Autodesk Inventor part; units mm, degrees
ref_plane "YZ Plane" through (0, 0, 0) normal (1, 0, 0) x (0, 1, 0)
ref_plane "XZ Plane" through (0, 0, 0) normal (0, 1, 0) x (-1, 0, 0)
ref_plane "XY Plane" through (0, 0, 0) normal (0, 0, 1) x (1, 0, 0)
sketch "Sketch1" plane through (0, 0, 0) normal (0, 1, 0) x (-1, 0, 0)
  line L0 (6, -1.25) -> (-6, -1.25)
  line L1 (-6, -1.25) -> (-6, 1.25)
  line L2 (-6, 1.25) -> (6, 1.25)
  line L3 (6, 1.25) -> (6, -1.25)
  line L4 (6, -1.25) -> (-6, 1.25) construction
  line L5 (-6, -1.25) -> (6, 1.25) construction
  point P0 (0, 0)
  dimension "d0" = 12
  dimension "d1" = 2.5
extrude "Extrusion1" add sketch "Sketch1" along normal blind 0.5
sketch "Sketch2" plane through (0, 0.5, 0) normal (0, 1, 0) x (1, 0, 0)
  circle A0 centre (-4.2565, 0) radius 0.75
  point P0 (0, 0)
  dimension "d4" = 1.5
extrude "Extrusion2" cut sketch "Sketch2" against normal blind 0.5
sketch "Sketch3" plane through (0, 0.5, 0) normal (0, 1, 0) x (1, 0, 0)
  circle A0 centre (-1.7501, 0) radius 0.75
  circle A1 centre (4.2419, 0) radius 0.75
  circle A2 centre (1.7477, 0) radius 0.75
  point P0 (0, 0)
  dimension "d7" = 1.5
  dimension "d8" = 1.5
  dimension "d9" = 1.5
extrude "Extrusion3" cut sketch "Sketch3" against normal blind 0.5 contours A0
sketch "Sketch7" plane through (0, 0.5, 0) normal (0, 1, 0) x (1, 0, 0)
  circle A0 centre (4.7487, 0) radius 0.15
  point P0 (0, 0)
  dimension "d21" = 0.3
extrude "Extrusion7" cut sketch "Sketch7" against normal blind 2
fillet "Fillet2" radius 0.5 1 edges at (6, 0.25, 1.25)
fillet "Fillet3" radius 0.5 1 edges at (6, 0.25, -1.25)
fillet "Fillet4" radius 0.5 1 edges at (-6, 0.25, 1.25)
fillet "Fillet5" radius 0.5 1 edges at (-6, 0.25, -1.25)
properties part number "stationary arm"
Work out the finished part from the listing and answer in its coordinate system (mm). Give positions to 0.01 mm unless a question says otherwise; leave off trailing zeros. Loops run counter-clockwise (first coordinate to the right, second up) from the corner with the lowest first, then second, coordinate; pieces in that order, holes last. Notation, with made-up numbers: (80.25, 14.5) - (100.25, 14.5) arc R26 cw to (100.25, 37.5) - close; hole circle Ø1 at (-30.75, 77). An arc over 180 degrees is marked (long way). Answer in a Markdown table with one row per item.
(1) A flat-ended cylindrical pin translates along its axis: pin 1 Ø1.2 at (x, z) = (-4.26, 0) entering from +Y. Find the tip coordinate at first contact, or state that the pin passes through.
Results list:
| item | result |
|---|---|
| pin 1 | passes through |
(2) Section A-A (x = 4.75) is taken. Give the vertices of the cut face in (y, z), and give its area (3 significant figures).
Results list:
| item | result |
|---|---|
| outline | (0, -1.25) - (0.5, -1.25) - (0.5, -0.15) - (0, -0.15) - close; (0, 0.15) - (0.5, 0.15) - (0.5, 1.25) - (0, 1.25) - close |
| area | 1.10 mm² |
(3) Consider L1, parallel to X at y = 0.45, z = 0; L2, parallel to X at y = 0.45, z = 0.6; L3, parallel to Z at x = -4, y = 0.2. Determine where each line is inside the solid, lowest interval first. Write a range as [from, to].
Results list:
| item | result |
|---|---|
| L1 | x = [-6, -5.01], [-3.51, -2.5], [-1, 4.6], [4.9, 6] |
| L2 | x = [-6, -4.71], [-3.81, -2.2], [-1.3, 6] |
| L3 | z = [-1.25, -0.7], [0.7, 1.25] |
(4) Section B-B (z = 0) is taken. Give the vertices of the cut face in (x, y), and give its area (3 significant figures).
Results list:
| item | result |
|---|---|
| outline | (-6, 0) - (-5.01, 0) - (-5.01, 0.5) - (-6, 0.5) - close; (-3.51, 0) - (-2.5, 0) - (-2.5, 0.5) - (-3.51, 0.5) - close; (-1, 0) - (4.6, 0) - (4.6, 0.5) - (-1, 0.5) - close; (4.9, 0) - (6, 0) - (6, 0.5) - (4.9, 0.5) - close |
| area | 4.35 mm² |
(5) For a pull along X with two mould halves and no side action, classify faces 1 (the face through (0, 0.5, 0)), 2 (the face through (-5.006, 0.254, -0.033)), 3 (the face through (-1.035, 0.254, -0.225)) as pulls with the +X half, pulls with the -X half, needs draft (parallel to the pull), parting line crosses it, or undercut.
Results list:
| item | result |
|---|---|
| face 1 | needs draft |
| face 2 | undercut |
| face 3 | undercut |
(6) Section C-C (y = 0.3) is taken. Give the vertices of the cut face in (x, z).
Results list:
| item | result |
|---|---|
| outline | (-6, -0.75) arc R0.5 ccw to (-5.5, -1.25) - (5.5, -1.25) arc R0.5 ccw to (6, -0.75) - (6, 0.75) arc R0.5 ccw to (5.5, 1.25) - (-5.5, 1.25) arc R0.5 ccw to (-6, 0.75) - close; hole circle Ø1.5 at (-4.26, 0); hole circle Ø1.5 at (-1.75, 0); hole circle Ø0.3 at (4.75, 0) |
